Job drawing, mm, ordinate dimensions from the low corner. One solid piece. A direction names the side the tool comes from. Coordinates: 2 decimals unless noted, no trailing zeros. Write each loop counter-clockwise with the first axis right and the second up, starting at its lowest first coordinate (ties: lowest second). Pieces come first, ordered by that corner, then holes. Notation, with made-up numbers: (-31.5, 32.25) -> (-20.5, 32.25) arc R32 cw to (-20.5, 65.25) -> close; hole circle Ø7 at (4.5, 33.25). An arc over 180 degrees is marked (long way). One line per question, with ' | ' between items. Start each with the question number.
Item 1: Saw through at D-D (y = 38.1). List the corners of the cut face in (x, z), and give its area (3 significant figures).
Item 2: Pin check, flat tips, straight feed: pin 1 (8 mm diameter, centred on y = 57, z = 16, fed in from +X); pin 2 (1 mm diameter, centred on y = 13.5, z = 23.5, fed in from -X); pin 3 (4 mm diameter, centred on x = 51.5, z = 27.5, fed in from +Y); pin 4 (8 mm diameter, centred on x = 26.94, y = 38.1, fed in from -Z). Stop position of each tip, or through.
Item 3: Saw through at C-C (y = 56). List the corners of the cut face in (x, z), and give its area (3 significant figures).
Item 4: Saw through at A-A (x = 53.34). List the corners of the cut face in (y, z).
Item 5: Probe probe 1 along Y at (x, z) = (53.34, 14.5); probe 2 along Y at (x, z) = (53, 13); probe 3 along Y at (x, z) = (30, 22.5) (1 decimal). List the from-to ranges inside material, lowest first. Write a range as [from, to].
Item 6: Saw through at B-B (z = 3). List the corners of the cut face in (x, y), and give its area (3 significant figures).
Item 7: 3-axis set-ups, long thin cutter, end or side, ignore diameter. For the marked faces 5 and 6: which of +Z, -Z, +X, -X, +Y, -Y reach the whole face in a straight line?
Item 8: Two-plate mould, pull along X, no slides. Class the marked faces 1, 2, 3 and 4: pulls with the +X half, pulls with the -X half, needs draft (parallel to the pull), parting line crosses it, or undercut.
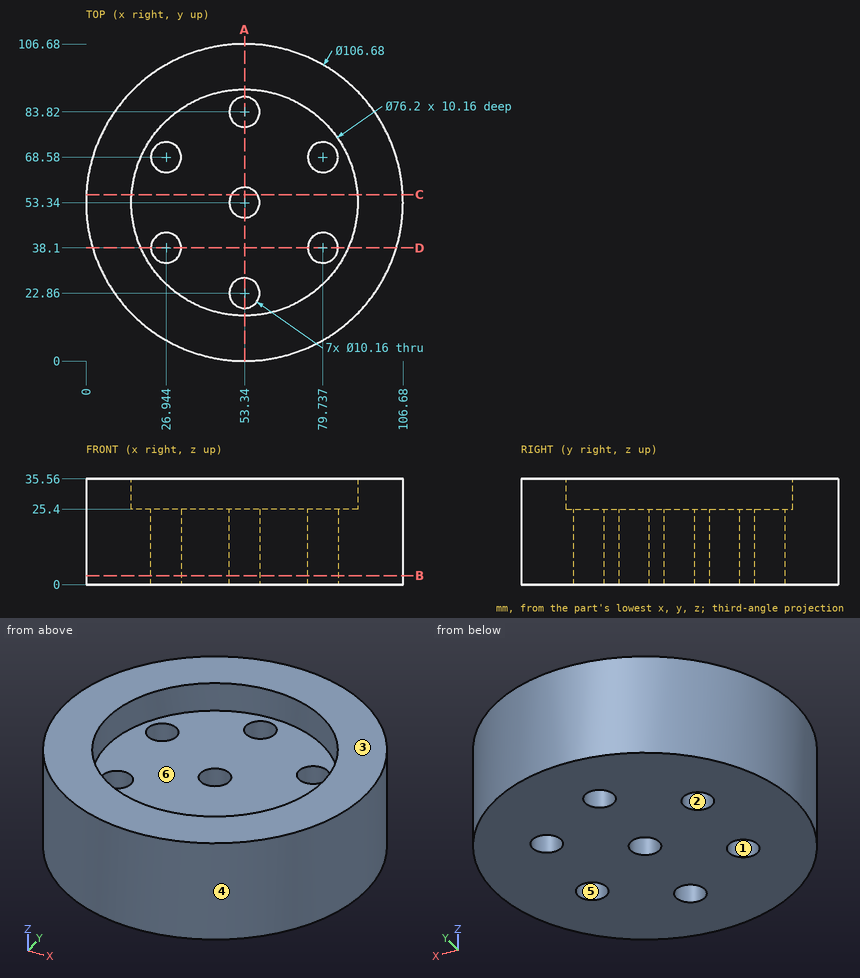
From the geometry:
1) outline: (2.22, 0) -> (21.86, 0) -> (21.86, 25.4) -> (18.42, 25.4) -> (18.42, 35.56) -> (2.22, 35.56) -> close; (32.02, 0) -> (74.66, 0) -> (74.66, 25.4) -> (32.02, 25.4) -> close; (84.82, 0) -> (104.46, 0) -> (104.46, 35.56) -> (88.26, 35.56) -> (88.26, 25.4) -> (84.82, 25.4) -> close | area: 2,410 mm2
2) pin 1: x = 106.68 | pin 2: x = 17.32 | pin 3: y = 106.68 | pin 4: through
3) outline: (0.07, 0) -> (49.01, 0) -> (49.01, 25.4) -> (15.33, 25.4) -> (15.33, 35.56) -> (0.07, 35.56) -> close; (57.67, 0) -> (106.61, 0) -> (106.61, 35.56) -> (91.35, 35.56) -> (91.35, 25.4) -> (57.67, 25.4) -> close | area: 2,800 mm2
4) outline: (0, 0) -> (17.78, 0) -> (17.78, 25.4) -> (15.24, 25.4) -> (15.24, 35.56) -> (0, 35.56) -> close; (27.94, 0) -> (48.26, 0) -> (48.26, 25.4) -> (27.94, 25.4) -> close; (58.42, 0) -> (78.74, 0) -> (78.74, 25.4) -> (58.42, 25.4) -> close; (88.9, 0) -> (106.68, 0) -> (106.68, 35.56) -> (91.44, 35.56) -> (91.44, 25.4) -> (88.9, 25.4) -> close
5) probe 1: [0, 17.78], [27.94, 48.26], [58.42, 78.74], [88.9, 106.68] | probe 2: [0, 17.79], [27.93, 48.27], [58.41, 78.75], [88.89, 106.68] | probe 3: [5.4, 34], [42.2, 64.5], [72.6, 101.3]
6) outline: circle Ø106.68 at (53.34, 53.34); hole circle Ø10.16 at (26.94, 38.1); hole circle Ø10.16 at (26.94, 68.58); hole circle Ø10.16 at (53.34, 22.86); hole circle Ø10.16 at (53.34, 53.34); hole circle Ø10.16 at (53.34, 83.82); hole circle Ø10.16 at (79.74, 38.1); hole circle Ø10.16 at (79.74, 68.58) | area: 8,370 mm2
7) face 5: +Z, -Z | face 6: +Z
8) face 1: undercut | face 2: undercut | face 3: needs draft | face 4: parting line crosses it
